Can you work these out from the drawing? Everything is in mm from the part's minimum corner. A direction names the side the tool comes from. Give positions to 0.01 mm unless a question says otherwise; leave off trailing zeros. Loops run counter-clockwise (first coordinate to the right, second up) from the corner with the lowest first, then second, coordinate; pieces in that order, holes last. Notation, with made-up numbers: (52.25, 61.25) -> (65.25, 61.25) arc R23 ccw to (65.25, 95.25) -> close; hole circle Ø4 at (29.25, 15). An arc over 180 degrees is marked (long way). Return JSON: item names as keys, results as strings. Group by question number.
Q1. Suppose I cut it at D-D, the plane y = 2.5. Please give me the cut outline in (x, z).
Q2. Thinking about a two-plate mould opening in Z: for the marked faces 1, 2 and 3, which applies, pulls with the +Z half, pulls with the -Z half, needs draft (parallel to the pull), parting line crosses it, or undercut?
Q3. Suppose I cut it at B-B, the plane z = 11. Please give me the cut outline in (x, y), and give its area (3 significant figures).
Q4. Which directions (+Z, -Z, +X, -X, +Y, -Y) give clear straight access to the entire face, cutting with the end or side of a thin tool? Please do the marked faces 4 and 5.
Q5. Suppose I cut it at C-C, the plane y = 14. Please give me the cut outline in (x, z), and give its area (3 significant figures).
Q6. Will these pins go through, and if not, where does the flat tip stop? pin 1 (6 mm diameter, centred on x = 4, z = 3, fed in from +Y); pin 2 (4 mm diameter, centred on x = 8, y = 3, fed in from -Z); pin 3 (6 mm diameter, centred on y = 9.5, z = 3.5, fed in from +X).
Q7. I need wall thicknesses on line 1 along Z through (x, y) = (11, 14.4); line 2 along Y through (x, z) = (5.75, 15.5); line 3 along Z through (x, y) = (11, 15.95). Which ranges of each line are inside material? Lowest first, please. Write a range as [from, to].
Q8. Suppose I cut it at A-A, the plane x = 11. Please give me the cut outline in (y, z).
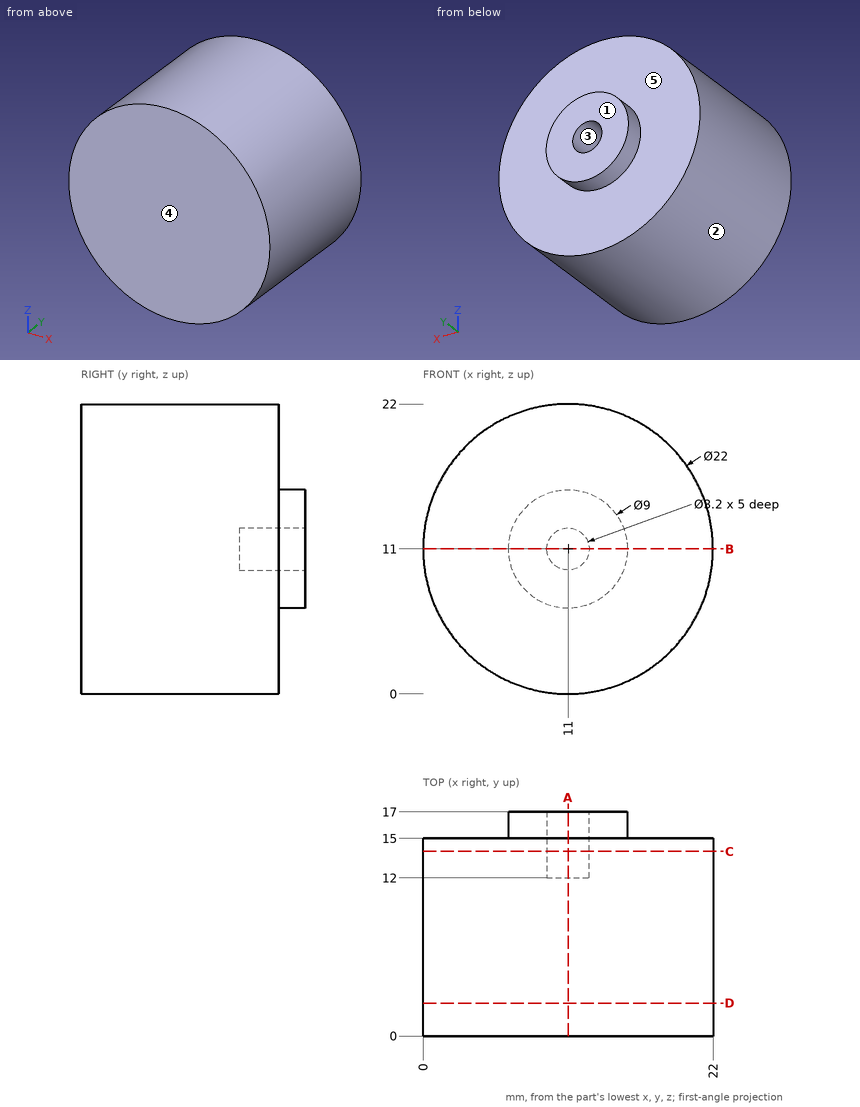
Ans:
{
 "1": {"outline": "circle Ø22 at (11, 11)"},
 "2": {"face 1": "needs draft", "face 2": "parting line crosses it", "face 3": "undercut"},
 "3": {"outline": "(0, 0) -> (22, 0) -> (22, 15) -> (15.5, 15) -> (15.5, 17) -> (12.6, 17) -> (12.6, 12) -> (9.4, 12) -> (9.4, 17) -> (6.5, 17) -> (6.5, 15) -> (0, 15) -> close", "area": "332 mm^2"},
 "4": {"face 4": "+Z, -Z, +X, -X, -Y", "face 5": "+Y"},
 "5": {"outline": "circle Ø22 at (11, 11); hole circle Ø3.2 at (11, 11)", "area": "372 mm^2"},
 "6": {"pin 1": "stops at y = 15", "pin 2": "stops at z = 0.05", "pin 3": "stops at x = 21.04"},
 "7": {"line 1": "z = [0, 9.4], [12.6, 22]", "line 2": "y = [0, 15]", "line 3": "z = [6.5, 9.4], [12.6, 15.5]"},
 "8": {"outline": "(0, 0) -> (15, 0) -> (15, 6.5) -> (17, 6.5) -> (17, 9.4) -> (12, 9.4) -> (12, 12.6) -> (17, 12.6) -> (17, 15.5) -> (15, 15.5) -> (15, 22) -> (0, 22) -> close"}
}
